The listing builds one solid part. Answer for the finished solid, in the listing's coordinates (mm). Round coordinates to 2 decimals unless told otherwise and drop trailing zeros. Write each loop counter-clockwise with the first axis right and the second up, starting at its lowest first coordinate (ties: lowest second). Pieces come first, ordered by that corner, then holes. Notation, with made-up numbers: (-1.75, 84.5) - (53.25, 84.5) arc R10 cw to (53.25, 89.5) - close; hole circle Ø2 at (21, -13.5). An arc over 180 degrees is marked (long way). Use a Markdown table: item, result. Add a question column.
1) Find the intervals of material crossed by probe 1 along X at (y, z) = (-201.5, 302); probe 2 along Z at (x, y) = (149, -202); probe 3 along X at (y, z) = (-270, 519.5), in increasing order. Write a range as from..to.
2) A cutting plane is placed at C-C (x = 16.5). Give the vertices of the cut face in (y, z), then the cut area to 3 significant figures.
3) Each of these flat-tipped pins is pushed along its axis until it touches: P1, Ø10, axis at x = 225, y = -169, coming from the -Z side; P2, Ø12, axis at y = -221, z = 278.5, coming from the -X side; P3, Ø10, axis at x = -15, y = -212, coming from the -Z side. Where does it stop, or does it pass through?
4) A cutting plane is placed at B-B (y = -129). Give the vertices of the cut face in (x, z), then the cut area to 3 significant figures.
5) A cutting plane is placed at A-A (z = 0). Give the vertices of the cut face in (x, y), then the cut area to 3 significant figures.
6) A cutting plane is placed at D-D (y = -81.5). Give the vertices of the cut face in (x, z), then the cut area to 3 significant figures.
7) Determine the mould class of faces 1 (the flat face through (300, -201, 511)), 2 (the flat face through (-1, 0, 1)), 3 (the flat face through (285, -201, 474)), 4 (the cylindrical face through (-6.503, -100.116, -29.287)) for opening direction X: +X half, -X half, draft (parallel to the pull), parting line (faces both ways), or undercut.
```python
from build123d import *

# Parameters (mm, degrees)
F0_R     = 30
F0_R_2   = 82.5
F5_DEPTH = 15
F6_R     = 82.5
F6_R_2   = 30
F7_DEPTH = 15


with BuildPart() as f4:
    # F4: sweep along a path in F1, F3
    with BuildLine(Plane.YZ) as f4_path:
        Line((0, 0), (-200, 0))
        Line((-200, 0), (-200, 510))
    with BuildLine(Plane.XZ.offset(200)) as f4_path_2:
        Line((0, 510), (300, 510))
    # F0 (on Front) → F4 (sweep)
    with BuildSketch(Plane.XZ):
        Circle(F0_R)
    sweep(path=f4_path.line + f4_path_2.line, transition=Transition.RIGHT)

    # F0 (on Front) → F5 (join)
    with BuildSketch(Plane.XZ):
        Circle(F0_R_2)
        Circle(F0_R, mode=Mode.SUBTRACT)
    extrude(amount=F5_DEPTH)

    # F6 (on face) → F7 (join)
    with BuildSketch(Plane.YZ.offset(300)):
        with Locations((-200, 510)):
            Circle(F6_R)
        with Locations((-200, 510)):
            Circle(F6_R_2, mode=Mode.SUBTRACT)
    extrude(amount=-F7_DEPTH)


solid = f4.part
```
Entries:
| question | item | result |
|---|---|---|
| 1 | probe 1 | x = -29.96..29.96 |
| 1 | probe 2 | z = 480.07..539.93 |
| 1 | probe 3 | x = 285..300 |
| 2 | outline | (-225.05, -25.05) - (-15, -25.05) - (-15, -80.83) - (0, -80.83) - (0, 80.83) - (-15, 80.83) - (-15, 25.05) - (-174.95, 25.05) - (-174.95, 493.5) arc R30 ccw (long way) to (-225.05, 493.5) - close |
| 2 | area | 38,800 mm² |
| 3 | P1 | stops at z = 495.03 |
| 3 | P2 | stops at x = -25.98 |
| 3 | P3 | stops at z = -28.28 |
| 4 | outline | circle Ø60 at (0, 0); (285, 467.99) - (300, 467.99) - (300, 552.01) - (285, 552.01) - close |
| 4 | area | 4,090 mm² |
| 5 | outline | (-82.5, -15) - (-30, -15) - (-30, -200) arc R30 ccw to (30, -200) - (30, -15) - (82.5, -15) - (82.5, 0) - (-82.5, 0) - close |
| 5 | area | 15,000 mm² |
| 6 | outline | circle Ø60 at (0, 0) |
| 6 | area | 2,830 mm² |
| 7 | face 1 | +X half |
| 7 | face 2 | draft |
| 7 | face 3 | undercut |
| 7 | face 4 | parting line |
